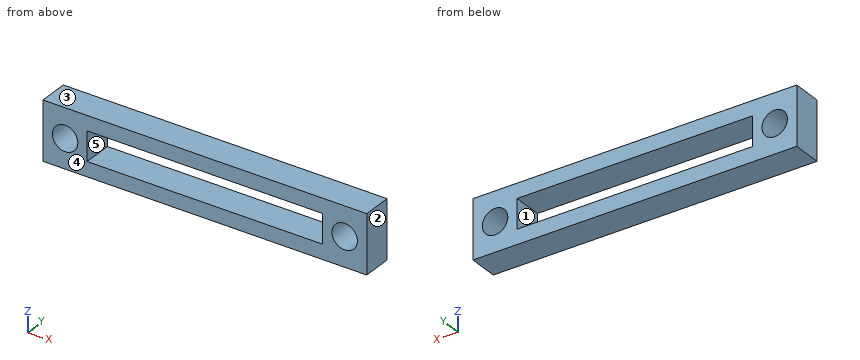
```python
from build123d import *

# Parameters (mm, degrees)
SKETCH1_W            = 69.85
SKETCH1_H            = 12.7
SKETCH1_W_2          = 50.8
SKETCH1_H_2          = 6.35
BOSS_EXTRUDE1_DEPTH  = 6.35
M5_CLEARANCE_HOLE1_D = 5.5


with BuildPart() as part:
    # Sketch1 → Boss-Extrude1 (new body)
    with BuildSketch(Plane(origin=(0, 0, 0), x_dir=(1, 0, 0), z_dir=(0, 1, 0))):
        Rectangle(SKETCH1_W, SKETCH1_H)
        Rectangle(SKETCH1_W_2, SKETCH1_H_2, mode=Mode.SUBTRACT)
    extrude(amount=BOSS_EXTRUDE1_DEPTH)

    # M5 Clearance Hole1 (through all)
    with Locations(Plane(origin=(0, 6.35, 0), x_dir=(1, 0, 0), z_dir=(0, 1, 0))):
        with Locations((-30.1625, 0)):
            m5_clearance_hole1 = Hole(M5_CLEARANCE_HOLE1_D / 2)

    # Mirror1: M5 Clearance Hole1 across plane
    add(m5_clearance_hole1.mirror(Plane(origin=(0, 0, 0), x_dir=(0, 0, 1), z_dir=(1, 0, 0))), mode=Mode.SUBTRACT)


solid = part.part
```
Geometry check sheet. Reference: the model listing, model coordinates, mm. Face numbers are marked on the shaded views. A direction names the side the tool comes from. Coordinates: 2 decimals unless noted, no trailing zeros. Loops run counter-clockwise (first coordinate to the right, second up) from the corner with the lowest first, then second, coordinate; pieces in that order, holes last. Notation, with made-up numbers: (14, 41) - (37, 41) arc R12 cw to (37, 59) - close; hole circle Ø10 at (-26.75, 68.5). An arc over 180 degrees is marked (long way). One line per item, written item: value. Start each with the question number.
(1) Mould release check, pull along X, two halves, no side actions. Record for the marked faces 1, 2 and 3: released by +X, released by -X, zero draft, split by the parting line, or undercut.
(2) Depth check by flat-ended pin: P1, Ø1.5, axis at x = -1, z = 4, coming from the -Y side; P2, Ø5, axis at x = -30.16, z = 0, coming from the +Y side. Enter the tip coordinate at first touch or a pass-through.
(3) Cross-section at B-B on x = -8.5. Enter the section's corners in (y, z) (3 decimals).
(4) Material ranges on line 1 (Z direction, x = -2.5, y = 5) (3 decimals); line 2 (X direction, y = 3.5, z = 0.5) (3 decimals); line 3 (X direction, y = 3.25, z = -2.5) (3 decimals), recorded low to high. Write a range as [from, to].
(5) Tool access check on the marked faces 4 and 5. Record the directions out of +Z, -Z, +X, -X, +Y, -Y that give a thin tool (end or side, any length) a straight path to the whole face; none if there is none.
(6) Cross-section at A-A on z = 0. Count the separate pieces of the cut face and the enclosed holes in it, plus the area to 3 significant figures.
Results below:
1. face 1: undercut
1. face 2: released by +X
1. face 3: zero draft
2. P1: stops at y = 0
2. P2: passes through
3. outline: (0, -6.35) - (6.35, -6.35) - (6.35, -3.175) - (0, -3.175) - close; (0, 3.175) - (6.35, 3.175) - (6.35, 6.35) - (0, 6.35) - close
4. line 1: z = [-6.35, -3.175], [3.175, 6.35]
4. line 2: x = [-34.925, -32.867], [-27.458, -25.4], [25.4, 27.458], [32.867, 34.925]
4. line 3: x = [-34.925, -31.308], [-29.017, -25.4], [25.4, 29.017], [31.308, 34.925]
5. face 4: +Z, -Z, +X, -X, -Y
5. face 5: +Y, -Y
6. separate pieces: 4
6. enclosed holes: 0
6. area: 51.1 mm2
